Source: CAD feature listing. Evaluate the final solid. Frame: model axes, mm. Face numbers are marked on the shaded views. Give positions to 0.01 mm unless a question says otherwise; leave off trailing zeros. Loops run counter-clockwise (first coordinate to the right, second up) from the corner with the lowest first, then second, coordinate; pieces in that order, holes last. Notation, with made-up numbers: (67.5, -2.75) -> (95.5, -2.75) arc R28 cw to (95.5, 25.25) -> close; hole circle Ø11 at (34, -25). An arc over 180 degrees is marked (long way). Answer as a JSON object with one key per item and string values. Group by question number.
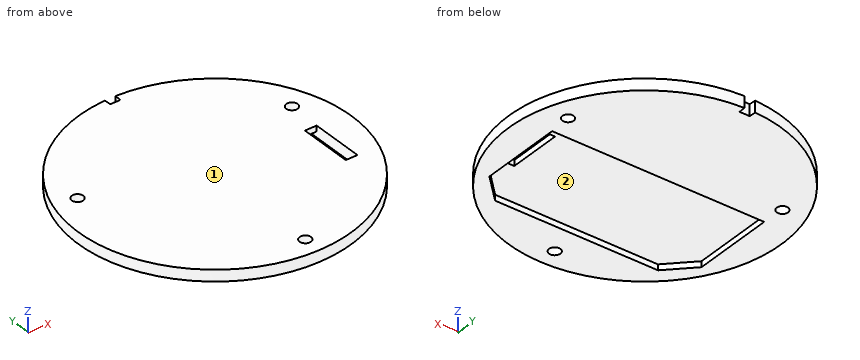
from build123d import *

# Parameters (mm, degrees)
SKETCH1_R           = 1.5
BOSS_EXTRUDE3_DEPTH = 3
BOSS_EXTRUDE4_DEPTH = 1.5


with BuildPart() as part:
    # Sketch1 → Boss-Extrude3 (new body)
    with BuildSketch(Plane.XY):
        with BuildLine():
            Line((-1.413353367, 35.972245305), (-1.342685699, 34.173633039))
            ThreePointArc((-1.342685699, 34.173633039), (0, 34.2), (1.342685699, 34.173633039))
            Line((1.342685699, 34.173633039), (1.413353367, 35.972245305))
            ThreePointArc((1.413353367, 35.972245305), (0, -36), (-1.413353367, 35.972245305))
        make_face()
        with Locations((28.3, 10.376069152)):
            Circle(SKETCH1_R, mode=Mode.SUBTRACT)
        with Locations((-28.3, 10.376069152)):
            Circle(SKETCH1_R, mode=Mode.SUBTRACT)
        with Locations((0, -31)):
            Circle(SKETCH1_R, mode=Mode.SUBTRACT)
        Polygon((-28, 4.5), (28, 4.5), (28, -17), (21.5, -23.5), (-21.5, -23.5), (-28, -17), align=None, mode=Mode.SUBTRACT)
    extrude(amount=-BOSS_EXTRUDE3_DEPTH)

    # Sketch1<9> → Boss-Extrude4 (add)
    with BuildSketch(Plane.XY):
        Polygon((28, 4.5), (0, 4.5), (0, -23.5), (21.5, -23.5), (28, -17), (28, -12.5), (24.9, -12.5), (24.9, 1.5), (28, 1.5), align=None)
        Polygon((0, -23.5), (0, 4.5), (-28, 4.5), (-28, -17), (-21.5, -23.5), align=None)
    extrude(amount=-BOSS_EXTRUDE4_DEPTH)


solid = part.part
(1) Section query A-A on y = 0. Return the cut outline in (x, z), plus the area to 3 significant figures.
(2) Mould query, pull axis Y, two halves, no side actions, for the marked faces 1 and 2. Classes: pulls with the +Y half, pulls with the -Y half, needs draft (parallel to the pull), parting line crosses it, or undercut.
(3) Material intervals for line 1 (Y direction, x = 0, z = -1.95); line 2 (Y direction, x = 0, z = -1.45); line 3 (Z direction, x = -26, y = -3), sorted ascending. Write a range as from..to.
(4) First-contact query: pin 1 (0.8 mm diameter, centred on x = 27, z = -1, fed in from +Y); pin 2 (0.8 mm diameter, centred on y = -7, z = -0.5, fed in from +X); pin 3 (1.8 mm diameter, centred on x = 28.3, y = 10.38, fed in from -Z); pin 4 (14 mm diameter, centred on x = 10, y = -12.5, fed in from -Z). Flat tips, straight axial feed; report the tip coordinate or a pass-through.
(5) Section query C-C on z = -2.45. Return the cut outline in (x, y), plus the area to 3 significant figures.
(6) Section query D-D on y = -31. Return the cut outline in (x, z).
(7) Section query B-B on x = 0. Return the cut outline in (y, z).
Result:
{
 "1": {"outline": "(-36, -3) -> (-28, -3) -> (-28, -1.5) -> (24.9, -1.5) -> (24.9, 0) -> (-36, 0) -> close; (28, -3) -> (36, -3) -> (36, 0) -> (28, 0) -> close", "area": "127 mm²"},
 "2": {"face 1": "needs draft", "face 2": "undercut"},
 "3": {"line 1": "-36..-32.5, -29.5..-23.5, 4.5..34.2", "line 2": "-36..-32.5, -29.5..34.2", "line 3": "-1.5..0"},
 "4": {"pin 1": "y = 24.26", "pin 2": "x = 35.39", "pin 3": "through", "pin 4": "z = -1.5"},
 "5": {"outline": "(-1.41, 35.97) arc R36 ccw (long way) to (1.41, 35.97) -> (1.34, 34.17) arc R34.2 ccw to (-1.34, 34.17) -> close; hole circle Ø3 at (-28.3, 10.38); hole (-28, -17) -> (-21.5, -23.5) -> (21.5, -23.5) -> (28, -17) -> (28, 4.5) -> (-28, 4.5) -> close; hole circle Ø3 at (0, -31); hole circle Ø3 at (28.3, 10.38)", "area": "2,520 mm²"},
 "6": {"outline": "(-18.3, -3) -> (-1.5, -3) -> (-1.5, 0) -> (-18.3, 0) -> close; (1.5, -3) -> (18.3, -3) -> (18.3, 0) -> (1.5, 0) -> close"},
 "7": {"outline": "(-36, -3) -> (-32.5, -3) -> (-32.5, 0) -> (-36, 0) -> close; (-29.5, -3) -> (-23.5, -3) -> (-23.5, -1.5) -> (4.5, -1.5) -> (4.5, -3) -> (34.2, -3) -> (34.2, 0) -> (-29.5, 0) -> close"}
}
